from build123d import *

# Parameters (mm, degrees)
SKETCH_1_R          = 1.5
EXTRUDE_1_DEPTH     = 4
SKETCH_2_R          = 1.5
EXTRUDE_2_DEPTH     = 16
CUT_EXTRUDE_4_DEPTH = 10
SKETCH_5_R          = 1.25
CUT_EXTRUDE_5_DEPTH = 8
SKETCH_6_R          = 1.5
EXTRUDE_3_DEPTH     = 30
CUT_EXTRUDE_6_DEPTH = 29
FILLET_2_R          = 2
SKETCH_11_R         = 1.5
EXTRUDE_4_DEPTH     = 4
FILLET_3_R          = 3
EXTRUDE_START       = -4
SKETCH_13_R         = 1.5
EXTRUDE_5_DEPTH     = 4


with BuildPart() as part:
    # 草图1 → 凸台-拉伸1 (new body)
    # profile 1 of 3: a face of its own
    with BuildSketch(Plane.XY):
        Polygon((-24, -8), (-13, -8), (-4, 1), (-8, 1), (-8, 8), (-24, 8), align=None)
        with Locations((-20, -5)):
            Circle(SKETCH_1_R, mode=Mode.SUBTRACT)
        with Locations((-20, 5)):
            Circle(SKETCH_1_R, mode=Mode.SUBTRACT)
    # profile 2 of 3: a face of its own
    with BuildSketch(Plane.XY):
        Polygon((-1, 8), (-1, 4), (8, 13), (8, 24), (-8, 24), (-8, 8), align=None)
        with Locations((-5, 20)):
            Circle(SKETCH_1_R, mode=Mode.SUBTRACT)
        with Locations((5, 20)):
            Circle(SKETCH_1_R, mode=Mode.SUBTRACT)
    # profile 3 of 3: a face of its own
    with BuildSketch(Plane.XY):
        Polygon((-8, 1), (-4, 1), (-1, 4), (-1, 8), (-8, 8), align=None)
        with Locations((-5, 5)):
            Circle(SKETCH_1_R, mode=Mode.SUBTRACT)
    extrude(amount=EXTRUDE_1_DEPTH)

    # 草图2 → 凸台-拉伸2 (add)
    with BuildSketch(Plane.XY.offset(4)):
        Polygon((-8, 17), (8, 17), (8, 13), (-13, -8), (-17, -8), (-17, 8), (-8, 8), align=None)
        with Locations((-5, 5)):
            Circle(SKETCH_2_R, mode=Mode.SUBTRACT)
    extrude(amount=EXTRUDE_2_DEPTH)

    # 草图4 → 切除-拉伸4 (cut)
    with BuildSketch(Plane(origin=(0, 0, 0), x_dir=(-1, 0, 0), z_dir=(0, 0, -1))):
        Polygon((-2.171572875, 10), (6, 10), (6, 15), (-6, 15), (-6, 13.828427125), align=None)
        Polygon((10.27723117, 6), (10.27723117, -2.448804045), (13.828427125, -6), (15, -6), (15, 6), align=None)
    extrude(amount=-CUT_EXTRUDE_4_DEPTH, mode=Mode.SUBTRACT)

    # 草图5 → 切除-拉伸5 (cut)
    with BuildSketch(Plane.XY.offset(20)):
        with Locations((-14, 5)):
            Circle(SKETCH_5_R)
        with Locations((-14, -5)):
            Circle(SKETCH_5_R)
        with Locations((-5, 14)):
            Circle(SKETCH_5_R)
        with Locations((5, 14)):
            Circle(SKETCH_5_R)
    extrude(amount=-CUT_EXTRUDE_5_DEPTH, mode=Mode.SUBTRACT)

    # 草图6 → 凸台-拉伸3 (add)
    with BuildSketch(Plane.XY.offset(20)):
        Polygon((-17, 8), (-8, 8), (-8, 17), (8, 17), (8, 13), (-13, -8), (-17, -8), align=None)
        with Locations((-14, 5)):
            Circle(SKETCH_6_R, mode=Mode.SUBTRACT)
        with Locations((-14, -5)):
            Circle(SKETCH_6_R, mode=Mode.SUBTRACT)
        with Locations((-5, 14)):
            Circle(SKETCH_6_R, mode=Mode.SUBTRACT)
        with Locations((5, 14)):
            Circle(SKETCH_6_R, mode=Mode.SUBTRACT)
    extrude(amount=EXTRUDE_3_DEPTH)

    # 草图7 → 切除-拉伸6 (cut)
    with BuildSketch(Plane.XY.offset(50)):
        with BuildLine():
            Line((-1, 15.5), (1, 15.5))
            ThreePointArc((1, 15.5), (2.5, 14), (1, 12.5))
            Line((1, 12.5), (-1, 12.5))
            ThreePointArc((-1, 12.5), (-2.5, 14), (-1, 15.5))
        make_face()
        with BuildLine():
            Line((-12.5, 1), (-12.5, -1))
            ThreePointArc((-12.5, -1), (-14, -2.5), (-15.5, -1))
            Line((-15.5, -1), (-15.5, 1))
            ThreePointArc((-15.5, 1), (-14, 2.5), (-12.5, 1))
        make_face()
    extrude(amount=-CUT_EXTRUDE_6_DEPTH, mode=Mode.SUBTRACT)

    # 圆角2
    fillet_2_edges = [part.edges().sort_by_distance(p)[0] for p in [
        (-13, -8, 25),
        (-24, -8, 2),
        (-24, 8, 2),
        (-8, 8, 25),
        (-8, 24, 2),
        (8, 24, 2),
        (8, 13, 25),
        (-17, 8, 27),
        (-17, -8, 27),
        (8, 17, 27),
        (-8, 17, 27),
    ]]
    fillet(fillet_2_edges, radius=FILLET_2_R)

    # 草图11 → 凸台-拉伸4 (add)
    with BuildSketch(Plane.XY.offset(50)):
        with BuildLine():
            Line((-13.828427125, -8), (-8, -8))
            Line((-8, -8), (-8, -24))
            Line((-8, -24), (8, -24))
            Line((8, -24), (8, -8))
            Line((8, -8), (24, -8))
            Line((24, -8), (24, 8))
            Line((24, 8), (8, 8))
            Line((8, 8), (8, 13.828427125))
            ThreePointArc((8, 13.828427125), (7.847759065, 13.06306026), (7.414213562, 12.414213562))
            Line((7.414213562, 12.414213562), (-12.414213562, -7.414213562))
            ThreePointArc((-12.414213562, -7.414213562), (-13.06306026, -7.847759065), (-13.828427125, -8))
        make_face()
        with Locations((21, 5)):
            Circle(SKETCH_11_R, mode=Mode.SUBTRACT)
        with Locations((21, -5)):
            Circle(SKETCH_11_R, mode=Mode.SUBTRACT)
        with Locations((11, -5)):
            Circle(SKETCH_11_R, mode=Mode.SUBTRACT)
        with Locations((11, 5)):
            Circle(SKETCH_11_R, mode=Mode.SUBTRACT)
        with Locations(Location((5, -21, 0), (0, 0, 180))):
            Circle(SKETCH_11_R, mode=Mode.SUBTRACT)
        with Locations(Location((-5, -21, 0), (0, 0, 180))):
            Circle(SKETCH_11_R, mode=Mode.SUBTRACT)
        with Locations(Location((-5, -11, 0), (0, 0, 180))):
            Circle(SKETCH_11_R, mode=Mode.SUBTRACT)
        with Locations(Location((5, -11, 0), (0, 0, 180))):
            Circle(SKETCH_11_R, mode=Mode.SUBTRACT)
    extrude(amount=-EXTRUDE_4_DEPTH)

    # 圆角3
    fillet_3_edges = [part.edges().sort_by_distance(p)[0] for p in [
        (-8, -24, 48),
        (-8, -8, 48),
        (8, 8, 48),
        (24, 8, 48),
        (24, -8, 48),
        (8, -8, 48),
        (8, -24, 48),
    ]]
    fillet(fillet_3_edges, radius=FILLET_3_R)

    # 草图13 → 凸台-拉伸5 (add)
    # profile 1 of 2: a face of its own
    with BuildSketch(Plane.XY.offset(50).offset(EXTRUDE_START)):
        with BuildLine():
            ThreePointArc((8, 22), (7.414213562, 23.414213562), (6, 24))
            Line((6, 24), (-6, 24))
            ThreePointArc((-6, 24), (-7.414213562, 23.414213562), (-8, 22))
            Line((-8, 22), (-8, 15))
            ThreePointArc((-8, 15), (-7.414213562, 16.414213562), (-6, 17))
            Line((-6, 17), (6, 17))
            ThreePointArc((6, 17), (7.414213562, 16.414213562), (8, 15))
            Line((8, 15), (8, 22))
        make_face()
        with Locations((-5, 20)):
            Circle(SKETCH_13_R, mode=Mode.SUBTRACT)
        with Locations((5, 20)):
            Circle(SKETCH_13_R, mode=Mode.SUBTRACT)
    # profile 2 of 2: a face of its own
    with BuildSketch(Plane.XY.offset(50).offset(EXTRUDE_START)):
        with BuildLine():
            ThreePointArc((-17, 6), (-16.414213562, 7.414213562), (-15, 8))
            Line((-15, 8), (-22, 8))
            ThreePointArc((-22, 8), (-23.414213562, 7.414213562), (-24, 6))
            Line((-24, 6), (-24, -6))
            ThreePointArc((-24, -6), (-23.414213562, -7.414213562), (-22, -8))
            Line((-22, -8), (-15, -8))
            ThreePointArc((-15, -8), (-16.414213562, -7.414213562), (-17, -6))
            Line((-17, -6), (-17, 6))
        make_face()
        with Locations((-20, -5)):
            Circle(SKETCH_13_R, mode=Mode.SUBTRACT)
        with Locations((-20, 5)):
            Circle(SKETCH_13_R, mode=Mode.SUBTRACT)
    extrude(amount=EXTRUDE_5_DEPTH)


solid = part.part
Part model, mm, in its own coordinate system. A direction names the side the tool comes from. Give positions to 0.01 mm unless a question says otherwise; leave off trailing zeros. Loops run counter-clockwise (first coordinate to the right, second up) from the corner with the lowest first, then second, coordinate; pieces in that order, holes last.
(1) Band-saw the part on B-B (z = 43). Write the cut outline in (x, y), and give its area (3 significant figures).
Return value:
outline: (-17, -6) arc R2 ccw to (-15, -8) - (-13.83, -8) arc R2 ccw to (-12.41, -7.41) - (7.41, 12.41) arc R2 ccw to (8, 13.83) - (8, 15) arc R2 ccw to (6, 17) - (-6, 17) arc R2 ccw to (-8, 15) - (-8, 10) arc R2 cw to (-10, 8) - (-15, 8) arc R2 ccw to (-17, 6) - close; hole circle Ø3 at (-14, -5); hole (-15.5, -1) arc R1.5 ccw to (-12.5, -1) - (-12.5, 1) arc R1.5 ccw to (-15.5, 1) - close; hole circle Ø3 at (-14, 5); hole circle Ø3 at (-5, 14); hole (-1, 12.5) - (1, 12.5) arc R1.5 ccw to (1, 15.5) - (-1, 15.5) arc R1.5 ccw to start; hole circle Ø3 at (5, 14)
area: 266 mm2
(2) 3-axis set-ups, long thin cutter, end or side, ignore diameter. For faces 1 (the cylindrical face through (-2.5, 14, 35.7)), 2 (the flat face through (-15, 0, 5)), 3 (the flat face through (8, 14.8, 26.7)), 4 (the cylindrical face through (-7.43, 16.4, 24.71)), 5 (the cylindrical face through (-23.4, 7.43, 47.97)): which of +Z, -Z, +X, -X, +Y, -Y reach the whole face in a straight line?
Return value:
face 1: +Z
face 2: -Z
face 3: +Z, -Z, +X, +Y
face 4: -X, +Y
face 5: +Z, -Z, -X, +Y
(3) Drill centre lines: line 1 along X through (y, z) = (-21, 47.55); line 2 along Y through (x, z) = (-14, 37); line 3 along Y through (x, z) = (-5, 28.5). Where is each one in solid material? Low to high.
Return value:
line 1: x = -8 to -6.5, -3.5 to 3.5, 6.5 to 8
line 2: y = -8 to -6.5, -3.5 to -2.5, 2.5 to 3.5, 6.5 to 8
line 3: y = 0 to 12.5, 15.5 to 17
(4) Pull direction Y, two halves, no side cores. Call faces 6 (the flat face through (16, 8, 48)), 7 (the flat face through (-24, 0, 2)), 8 (the flat face through (-6, 12, 5)), 9 (the cylindrical face through (23.14, -7.1, 47.97)): pulls with the +Y half, pulls with the -Y half, needs draft (parallel to the pull), parting line crosses it, or undercut.
Return value:
face 6: pulls with the +Y half
face 7: needs draft
face 8: undercut
face 9: pulls with the -Y half
(5) Pin check, flat tips, straight feed: pin 1 (13 mm diameter, centred on x = 2.5, z = 20.5, fed in from +Y); pin 2 (1 mm diameter, centred on y = 6.5, z = 34, fed in from +X); pin 3 (4 mm diameter, centred on x = -3.5, y = -7, fed in from -Z); pin 4 (3 mm diameter, centred on x = -4.5, y = 14.5, fed in from +Z). Stop position of each tip, or through.
Return value:
pin 1: stops at y = 17
pin 2: stops at x = 2
pin 3: stops at z = 46
pin 4: stops at z = 50
(6) Band-saw the part on D-D (z = 13). Write the cut outline in (x, y), and give its area (3 significant figures).
Return value:
outline: (-17, -6) arc R2 ccw to (-15, -8) - (-13.83, -8) arc R2 ccw to (-12.41, -7.41) - (7.41, 12.41) arc R2 ccw to (8, 13.83) - (8, 15) arc R2 ccw to (6, 17) - (-6, 17) arc R2 ccw to (-8, 15) - (-8, 10) arc R2 cw to (-10, 8) - (-15, 8) arc R2 ccw to (-17, 6) - close; hole circle Ø2.5 at (-14, -5); hole circle Ø2.5 at (-14, 5); hole circle Ø3 at (-5, 5); hole circle Ø2.5 at (-5, 14); hole circle Ø2.5 at (5, 14)
area: 294 mm2
(7) Band-saw the part on A-A (x = -20). Write the cut outline in (y, z), and give its area (3 significant figures).
Return value:
outline: (-8, 0) - (-6.5, 0) - (-6.5, 4) - (-8, 4) - close; (-8, 46) - (-6.5, 46) - (-6.5, 50) - (-8, 50) - close; (-3.5, 0) - (3.5, 0) - (3.5, 4) - (-3.5, 4) - close; (-3.5, 46) - (3.5, 46) - (3.5, 50) - (-3.5, 50) - close; (6.5, 0) - (8, 0) - (8, 4) - (6.5, 4) - close; (6.5, 46) - (8, 46) - (8, 50) - (6.5, 50) - close
area: 80.0 mm2
